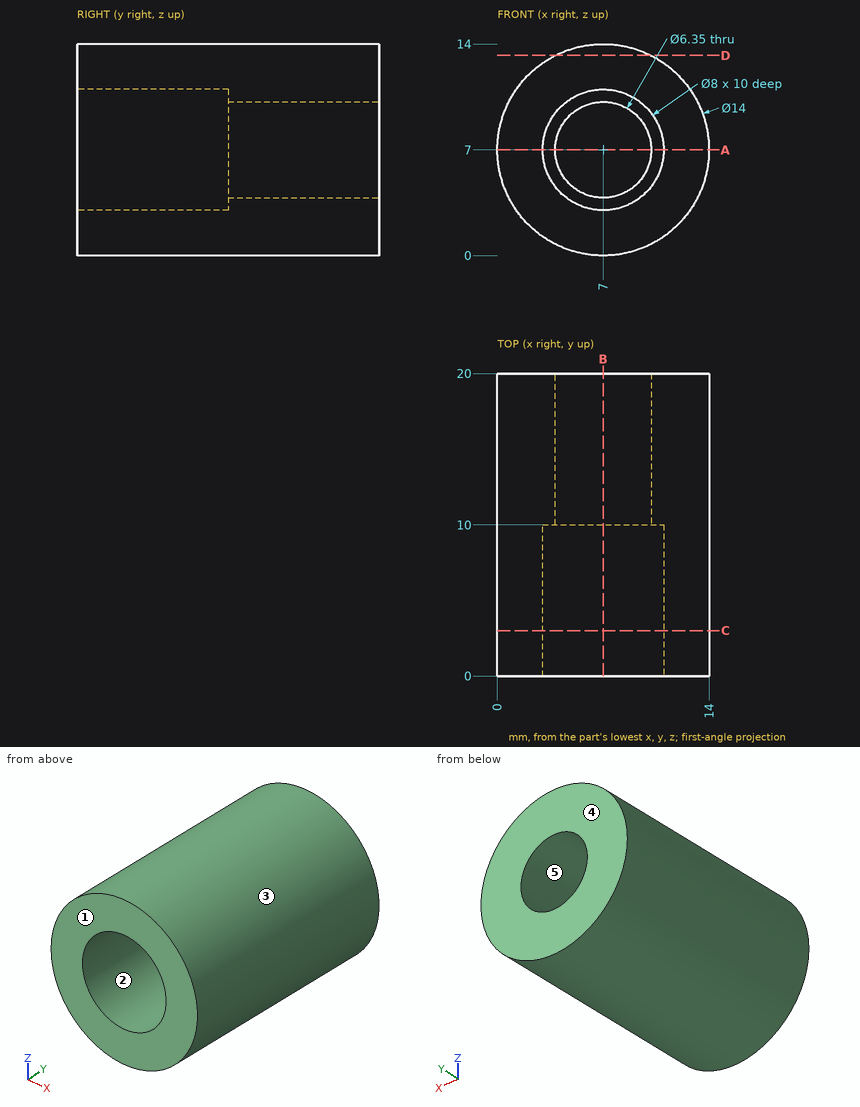
Could you check a few things on this drawing? It's one solid part, dimensions in mm from its lowest x, y, z. A direction names the side the tool comes from. Coordinates: 2 decimals unless noted, no trailing zeros. Loops run counter-clockwise (first coordinate to the right, second up) from the corner with the lowest first, then second, coordinate; pieces in that order, holes last. Notation, with made-up numbers: (22.25, -7) - (81.25, -7) arc R15 cw to (81.25, 17) - close; hole circle Ø3 at (54.25, 32). An arc over 180 degrees is marked (long way). Return JSON: item names as keys, results as strings. Group by question number.
Item 1: If we section it at A-A on z = 7: Write out the boundary of the cut face in (x, y) (3 decimals).
Item 2: If we section it at B-B on x = 7: Write out the boundary of the cut face in (y, z) (3 decimals).
Item 3: We'd pull the mould along X, two halves only. Please class the marked faces 3, 4 and 5: +X half, -X half, draft (parallel to the pull), parting line (faces both ways), or undercut.
Item 4: If we section it at D-D on z = 13.25: Write out the boundary of the cut face in (x, y), and give its area (3 significant figures).
Item 5: If we section it at C-C on y = 3: Write out the boundary of the cut face in (x, z).
Item 6: On a 3-axis mill with a long thin cutter (end or side, diameter ignored), from which of +Z, -Z, +X, -X, +Y, -Y can I reach the whole of each face in a straight line? I mean the marked faces 1 and 2. Say none if no direction works.
Item 7: I need wall thicknesses on line 1 (Z direction, x = 7, y = 3.5); line 2 (Z direction, x = 7, y = 17) (3 decimals); line 3 (Y direction, x = 3.5, z = 7.25). Which ranges of each line are inside material? Lowest first, please. Write a range as from..to.
Item 8: Will these pins go through, and if not, where does the flat tip stop? P1, Ø3, axis at x = 6, z = 4, coming from the -Y side; P2, Ø1.5, axis at x = 12, y = 9.5, coming from the +Z side; P3, Ø2, axis at y = 6.5, z = 5, coming from the -X side; P4, Ø1, axis at y = 10.5, z = 5, coming from the +X side.
Calculated:
{
 "1": {"outline": "(0, 0) - (3, 0) - (3, 10) - (3.825, 10) - (3.825, 20) - (0, 20) - close; (10.175, 10) - (11, 10) - (11, 0) - (14, 0) - (14, 20) - (10.175, 20) - close"},
 "2": {"outline": "(0, 0) - (20, 0) - (20, 3.825) - (10, 3.825) - (10, 3) - (0, 3) - close; (0, 11) - (10, 11) - (10, 10.175) - (20, 10.175) - (20, 14) - (0, 14) - close"},
 "3": {"face 3": "parting line", "face 4": "draft", "face 5": "undercut"},
 "4": {"outline": "(3.85, 0) - (10.15, 0) - (10.15, 20) - (3.85, 20) - close", "area": "126 mm^2"},
 "5": {"outline": "circle Ø14 at (7, 7); hole circle Ø8 at (7, 7)"},
 "6": {"face 1": "+Z, -Z, +X, -X, -Y", "face 2": "-Y"},
 "7": {"line 1": "z = 0..3, 11..14", "line 2": "z = 0..3.825, 10.175..14", "line 3": "y = 10..20"},
 "8": {"P1": "stops at y = 0", "P2": "stops at z = 12.56", "P3": "stops at x = 0.07", "P4": "stops at x = 13.84"}
}
